Source: CAD feature listing. Evaluate the final solid. Frame: model axes, mm. A direction names the side the tool comes from. Coordinates: 2 decimals unless noted, no trailing zeros. Write each loop counter-clockwise with the first axis right and the second up, starting at its lowest first coordinate (ties: lowest second). Pieces come first, ordered by that corner, then holes. Notation, with made-up numbers: (-19, -18.75) -> (-13, -18.75) arc R17 cw to (-13, 3.25) -> close; hole circle Ø10 at (-0.75, 78.5). An arc over 180 degrees is marked (long way). One line per item, written item: value. Start each with the question number.
1. Section query A-A, the plane y = -27.5. Output: boundary loops of the cut face in (x, z), and give its area (3 significant figures).
2. Access query for faces 1 (the flat face through (20.499, -27, 37)), 2 (the flat face through (-19, -23, 32.5)), 3 (the flat face through (-20.501, -27, 36)), 4 (the flat face through (17, -20, 12)). Directions: +Z, -Z, +X, -X, +Y, -Y. A direction counts if a zero-diameter tool reaches every point of the face in a straight line with its end or side. Return the directions, or none.
3. Section query B-B, the plane x = -30.8. Output: boundary loops of the cut face in (y, z), and give its area (3 significant figures).
4. Mould query, pull axis Z, two halves, no side actions, for faces 5 (the flat face through (15.52, -13.35, 11.54)), 6 (the cylindrical face through (13, -28, 9)), 7 (the cylindrical face through (32.2, -24.4, 2)). Classes: released by +Z, released by -Z, zero draft, split by the parting line, or undercut.
5. Section query C-C, the plane y = -23.35. Output: boundary loops of the cut face in (x, z).
6. First-contact query: P1, Ø3.5, axis at x = -19, y = -24, coming from the +Z side; P2, Ø10, axis at y = -16.5, z = 12, coming from the -X side; P3, Ø5, axis at x = -20, y = -12, coming from the -Z side; P4, Ø3, axis at x = 30.8, y = -8.65, coming from the -Z side. Flat tips, straight axial feed; report the tip coordinate or a pass-through.
7. Section query D-D, the plane z = 20. Output: boundary loops of the cut face in (x, y).
8. Line query: line 1 (X direction, y = -26.7, z = 7.5); line 2 (X direction, y = -27.1, z = 40.5); line 3 (Y direction, x = -20.15, z = 2.55). Output: solid intervals per line, ascending.
from build123d import *

# Parameters (mm, degrees)
SKETCH_1_W          = 34
SKETCH_1_H          = 51
EXTRUDE_1_DEPTH     = 4
SKETCH_5_W          = 34
SKETCH_5_H          = 15
EXTRUDE_2_DEPTH     = 4
SKETCH_6_R          = 1.5
CUT_EXTRUDE_3_DEPTH = 4
SKETCH_12_W         = 34
SKETCH_12_H         = 4
CUT_EXTRUDE_5_DEPTH = 5
SKETCH_13_W         = 34
SKETCH_13_H         = 4
CUT_EXTRUDE_6_DEPTH = 7
SKETCH_14_W         = 34
SKETCH_14_H         = 4
EXTRUDE_3_DEPTH     = 33
SKETCH_15_R         = 1.75
CUT_EXTRUDE_7_DEPTH = 44
EXTRUDE_4_DEPTH     = 3
EXTRUDE_5_DEPTH     = 3
SKETCH_18_R         = 1.75
EXTRUDE_6_DEPTH     = 4
EXTRUDE_7_DEPTH     = 5
SKETCH_20_W         = 4
SKETCH_20_H         = 43
EXTRUDE_8_DEPTH     = 20
SKETCH_21_W         = 4
SKETCH_21_H         = 43
EXTRUDE_9_DEPTH     = 20
SKETCH_22_W         = 74
SKETCH_22_H         = 4
CUT_EXTRUDE_8_DEPTH = 16
SKETCH_23_R         = 1.75
CUT_EXTRUDE_9_DEPTH = 16
FILLET_1_R          = 5


with BuildPart() as part:
    # 草图1 → 凸台-拉伸1 (new body)
    with BuildSketch(Plane.XY):
        Rectangle(SKETCH_1_W, SKETCH_1_H)
    extrude(amount=EXTRUDE_1_DEPTH)

    # 草图5 → 凸台-拉伸2 (add)
    with BuildSketch(Plane.XZ.offset(25.5)):
        with Locations((0, 7.5)):
            Rectangle(SKETCH_5_W, SKETCH_5_H)
    extrude(amount=EXTRUDE_2_DEPTH)

    # 草图6 → 切除-拉伸3 (cut)
    with BuildSketch(Plane.XZ.offset(29.5)):
        with Locations(Location((13, 7.5, 0), (0, 0, 270))):
            Circle(SKETCH_6_R)
        with Locations(Location((-13, 7.5, 0), (0, 0, 90))):
            Circle(SKETCH_6_R)
    extrude(amount=-CUT_EXTRUDE_3_DEPTH, mode=Mode.SUBTRACT)

    # 草图12 → 切除-拉伸5 (cut)
    with BuildSketch(Plane(origin=(0, 25.5, 0), x_dir=(1, 0, 0), z_dir=(0, 1, 0))):
        with Locations((0, -2)):
            Rectangle(SKETCH_12_W, SKETCH_12_H)
    extrude(amount=-CUT_EXTRUDE_5_DEPTH, mode=Mode.SUBTRACT)

    # 草图13 → 切除-拉伸6 (cut)
    with BuildSketch(Plane(origin=(0, 20.5, 0), x_dir=(1, 0, 0), z_dir=(0, 1, 0))):
        with Locations((0, -2)):
            Rectangle(SKETCH_13_W, SKETCH_13_H)
    extrude(amount=-CUT_EXTRUDE_6_DEPTH, mode=Mode.SUBTRACT)

    # 草图14 → 凸台-拉伸3 (add)
    with BuildSketch(Plane.XY.offset(15)):
        with Locations((0, -27.5)):
            Rectangle(SKETCH_14_W, SKETCH_14_H)
    extrude(amount=EXTRUDE_3_DEPTH)

    # 草图15 → 切除-拉伸7 (cut)
    with BuildSketch(Plane(origin=(0, -25.5, 0), x_dir=(1, 0, 0), z_dir=(0, 1, 0))):
        with Locations(Location((13, -40.5, 0), (0, 0, 270))):
            Circle(SKETCH_15_R)
        with Locations(Location((-13, -40.5, 0), (0, 0, 270))):
            Circle(SKETCH_15_R)
    extrude(amount=-CUT_EXTRUDE_7_DEPTH, mode=Mode.SUBTRACT)

    # 草图16 → 凸台-拉伸4 (add)
    with BuildSketch(Plane.ZY.offset(17)):
        Polygon((4, -25.5), (4, -6), (24, -25.5), align=None)
    extrude(amount=-EXTRUDE_4_DEPTH)

    # 草图17 → 凸台-拉伸5 (add)
    with BuildSketch(Plane(origin=(17, 0, 0), x_dir=(0, 0, -1), z_dir=(1, 0, 0))):
        Polygon((-24, -25.5), (-4, -6), (-4, -25.5), align=None)
    extrude(amount=-EXTRUDE_5_DEPTH)

    # 草图18 → 凸台-拉伸6 (add)
    with BuildSketch(Plane(origin=(0, -25.5, 0), x_dir=(1, 0, 0), z_dir=(0, 1, 0))):
        with BuildLine():
            Line((20.499000769, -32.499999751), (17, -24))
            Line((17, -24), (-17, -24))
            Line((-17, -24), (-20.500999231, -32.499999751))
            Line((-20.500999231, -32.499999751), (-20.500999231, -40.499999751))
            ThreePointArc((-20.500999231, -40.499999751), (-17.718513652, -47.217514172), (-11.000999231, -49.999999751))
            Line((-11.000999231, -49.999999751), (10.999000769, -49.999999751))
            ThreePointArc((10.999000769, -49.999999751), (17.71651519, -47.217514172), (20.499000769, -40.499999751))
            Line((20.499000769, -40.499999751), (20.499000769, -32.499999751))
        make_face()
        with Locations(Location((-13, -40.5, 0), (0, 0, 270))):
            Circle(SKETCH_18_R, mode=Mode.SUBTRACT)
        with Locations(Location((13, -40.5, 0), (0, 0, 270))):
            Circle(SKETCH_18_R, mode=Mode.SUBTRACT)
    extrude(amount=-EXTRUDE_6_DEPTH)

    # 草图19 → 凸台-拉伸7 (add)
    with BuildSketch(Plane(origin=(0, -25.5, 0), x_dir=(1, 0, 0), z_dir=(0, 1, 0))):
        Polygon((-20.500999231, -32.499999751), (-17.500999231, -32.499999751), (-14, -24), (-14, -16), (-17, -16), (-17, -24), align=None)
        Polygon((17, -24), (20.499000769, -32.499999751), (17.499000769, -32.499999751), (14, -24), (14, -16), (17, -16), align=None)
    extrude(amount=EXTRUDE_7_DEPTH)

    # 草图20 → 凸台-拉伸8 (add)
    with BuildSketch(Plane(origin=(17, 0, 0), x_dir=(0, 0, -1), z_dir=(1, 0, 0))):
        with Locations((-2, -8)):
            Rectangle(SKETCH_20_W, SKETCH_20_H)
    extrude(amount=EXTRUDE_8_DEPTH)

    # 草图21 → 凸台-拉伸9 (add)
    with BuildSketch(Plane.ZY.offset(17)):
        with Locations((2, -8)):
            Rectangle(SKETCH_21_W, SKETCH_21_H)
    extrude(amount=EXTRUDE_9_DEPTH)

    # 草图22 → 切除-拉伸8 (cut)
    with BuildSketch(Plane(origin=(0, 13.5, 0), x_dir=(1, 0, 0), z_dir=(0, 1, 0))):
        with Locations((0, -2)):
            Rectangle(SKETCH_22_W, SKETCH_22_H)
    extrude(amount=-CUT_EXTRUDE_8_DEPTH, mode=Mode.SUBTRACT)

    # 草图23 → 切除-拉伸9 (cut)
    with BuildSketch(Plane(origin=(0, 0, 0), x_dir=(-1, 0, 0), z_dir=(0, 0, -1))):
        with Locations((30.8, -8.65)):
            Circle(SKETCH_23_R)
        with Locations((-30.8, -8.65)):
            Circle(SKETCH_23_R)
        with Locations((-30.8, -23.35)):
            Circle(SKETCH_23_R)
        with Locations((20.15, -23.35)):
            Circle(SKETCH_23_R)
    extrude(amount=-CUT_EXTRUDE_9_DEPTH, mode=Mode.SUBTRACT)

    # 圆角1
    fillet_1_edges = [part.edges().sort_by_distance(p)[0] for p in [
        (37, -29.5, 2),
        (-37, -29.5, 2),
        (-37, -2.5, 2),
        (37, -2.5, 2),
    ]]
    fillet(fillet_1_edges, radius=FILLET_1_R)


solid = part.part
Computed values:
1. outline: (-36, 0) -> (36, 0) -> (36, 4) -> (17, 4) -> (17, 24) -> (20.5, 32.5) -> (20.5, 40.5) arc R9.5 ccw to (17, 47.86) -> (17, 48) -> (16.83, 48) arc R9.5 ccw to (11, 50) -> (-11, 50) arc R9.5 ccw to (-16.83, 48) -> (-17, 48) -> (-17, 47.87) arc R9.5 ccw to (-20.5, 40.5) -> (-20.5, 32.5) -> (-17, 24) -> (-17, 4) -> (-36, 4) -> close; hole circle Ø3.5 at (-13, 40.5); hole circle Ø3 at (-13, 7.5); hole circle Ø3.5 at (13, 40.5); hole circle Ø3 at (13, 7.5)
1. area: 1,930 mm²
2. face 1: +Z, +X, +Y, -Y
2. face 2: +Z, +X, -X, +Y
2. face 3: +Z, -X, +Y, -Y
2. face 4: +X, +Y, -Y
3. outline: (-29.5, 0) -> (-10.4, 0) -> (-10.4, 4) -> (-29.5, 4) -> close; (-6.9, 0) -> (-2.5, 0) -> (-2.5, 4) -> (-6.9, 4) -> close
3. area: 94.0 mm²
4. face 5: released by +Z
4. face 6: undercut
4. face 7: zero draft
5. outline: (-37, 0) -> (-21.9, 0) -> (-21.9, 4) -> (-37, 4) -> close; (-20.5, 32.5) -> (-17, 24) -> (-17, 4) -> (-18.4, 4) -> (-18.4, 0) -> (29.05, 0) -> (29.05, 4) -> (17, 4) -> (17, 24) -> (20.5, 32.5) -> (17.5, 32.5) -> (14, 24) -> (14, 4) -> (-14, 4) -> (-14, 24) -> (-17.5, 32.5) -> close; (32.55, 0) -> (37, 0) -> (37, 4) -> (32.55, 4) -> close
6. P1: stops at z = 46.81
6. P2: stops at x = -17
6. P3: stops at z = 0
6. P4: passes through
7. outline: (-17, -29.5) -> (17, -29.5) -> (17, -20.5) -> (14, -20.5) -> (14, -25.5) -> (-14, -25.5) -> (-14, -20.5) -> (-17, -20.5) -> close
8. line 1: x = -17 to -14.5, -11.5 to 11.5, 14.5 to 17
8. line 2: x = -20.5 to -14.75, -11.25 to 11.25, 14.75 to 20.5
8. line 3: y = -29.5 to -25.1, -21.6 to -2.5
